```python
from build123d import *

# Parameters (mm, degrees)
F1_DEPTH = 5.588
F3_DEPTH = 7.62
F4_R     = 3.175
F5_DEPTH = 12.7
F6_R     = 1.27
F7_DEPTH = 8.128


with BuildPart() as f1:
    # F0 (on Front) → F1 (new body)
    with BuildSketch(Plane.XZ):
        with BuildLine():
            Line((12.7, -41.275), (12.7, 41.275))
            ThreePointArc((12.7, 41.275), (0, 53.975), (-12.7, 41.275))
            Line((-12.7, 41.275), (-12.7, -41.275))
            ThreePointArc((-12.7, -41.275), (0, -53.975), (12.7, -41.275))
        make_face()
    extrude(amount=F1_DEPTH)

    # F2 (on face) → F3 (join)
    with BuildSketch(Plane(origin=(0, 0, 0), x_dir=(-1, 0, 0), z_dir=(0, 1, 0))):
        with BuildLine():
            ThreePointArc((4.445, 34.3189235197), (7.2401139494, 37.309426271), (8.255, 41.275))
            ThreePointArc((8.255, 41.275), (-3.965573729, 48.5151139494), (-4.445, 34.3189235197))
            ThreePointArc((-4.445, 34.3189235197), (0, 33.02), (4.445, 34.3189235197))
        make_face()
        with BuildLine():
            ThreePointArc((4.445, 34.3189235197), (0, 33.02), (-4.445, 34.3189235197))
            Line((-4.445, 34.3189235197), (-4.445, 3.7810764803))
            ThreePointArc((-4.445, 3.7810764803), (0, 5.08), (4.445, 3.7810764803))
            Line((4.445, 3.7810764803), (4.445, 34.3189235197))
        make_face()
        with BuildLine():
            ThreePointArc((4.445, 3.7810764803), (0, 5.08), (-4.445, 3.7810764803))
            ThreePointArc((-4.445, 3.7810764803), (-8.2238434682, -3.89153584), (-3.175, -10.795))
            ThreePointArc((-3.175, -10.795), (0, -10.16), (3.175, -10.795))
            ThreePointArc((3.175, -10.795), (6.8685751798, -7.7540501198), (8.255, -3.175))
            ThreePointArc((8.255, -3.175), (7.2401139494, 0.790573729), (4.445, 3.7810764803))
        make_face()
        with BuildLine():
            ThreePointArc((3.175, -10.795), (0, -11.43), (-3.175, -10.795))
            ThreePointArc((-3.175, -10.795), (-8.2238434682, -17.69846416), (-4.445, -25.3710764803))
            ThreePointArc((-4.445, -25.3710764803), (0, -26.67), (4.445, -25.3710764803))
            ThreePointArc((4.445, -25.3710764803), (7.2401139494, -22.380573729), (8.255, -18.415))
            ThreePointArc((8.255, -18.415), (6.8685751798, -13.8359498802), (3.175, -10.795))
        make_face()
        with BuildLine():
            ThreePointArc((3.175, -10.795), (0, -10.16), (-3.175, -10.795))
            ThreePointArc((-3.175, -10.795), (0, -11.43), (3.175, -10.795))
        make_face()
        with BuildLine():
            ThreePointArc((4.445, -25.3710764803), (0, -26.67), (-4.445, -25.3710764803))
            Line((-4.445, -25.3710764803), (-4.445, -34.3189235197))
            ThreePointArc((-4.445, -34.3189235197), (0, -33.02), (4.445, -34.3189235197))
            Line((4.445, -34.3189235197), (4.445, -25.3710764803))
        make_face()
        with BuildLine():
            ThreePointArc((4.445, -34.3189235197), (0, -33.02), (-4.445, -34.3189235197))
            ThreePointArc((-4.445, -34.3189235197), (-3.965573729, -48.5151139494), (8.255, -41.275))
            ThreePointArc((8.255, -41.275), (7.2401139494, -37.309426271), (4.445, -34.3189235197))
        make_face()
    extrude(amount=F3_DEPTH)

    # F4 (on face) → F5 (join)
    with BuildSketch(Plane.XZ.offset(5.588)):
        with Locations((0, -41.275)):
            Circle(F4_R)
        with Locations((0, 41.275)):
            Circle(F4_R)
        with Locations((0, -3.175)):
            Circle(F4_R)
        with Locations((0, -18.415)):
            Circle(F4_R)
    extrude(amount=F5_DEPTH)

    # F6 (on face) → F7 (join)
    with BuildSketch(Plane.XZ.offset(18.288)):
        with Locations((0, 41.275)):
            Circle(F6_R)
        with Locations((0, -3.175)):
            Circle(F6_R)
        with Locations((0, -18.415)):
            Circle(F6_R)
        with Locations((0, -41.275)):
            Circle(F6_R)
    extrude(amount=F7_DEPTH)


solid = f1.part
```
Build history of the part. All positions in model axes, mm. A direction names the side the tool comes from. Give positions to 0.01 mm unless a question says otherwise; leave off trailing zeros. Loops run counter-clockwise (first coordinate to the right, second up) from the corner with the lowest first, then second, coordinate; pieces in that order, holes last.
1) Band-saw the part on D-D on y = -23. List the corners of the cut face in (x, z) (3 decimals), then the cut area to 3 significant figures.
Values follow:
outline: circle Ø2.54 at (0, -41.275); circle Ø2.54 at (0, -18.415); circle Ø2.54 at (0, -3.175); circle Ø2.54 at (0, 41.275)
area: 20.3 mm2
2) Band-saw the part on C-C on x = -10.25. List the corners of the cut face in (y, z), then the cut area to 3 significant figures.
Values follow:
outline: (-5.59, -48.77) - (0, -48.77) - (0, 48.77) - (-5.59, 48.77) - close
area: 545 mm2
3) Drop flat-ended pins along their axis: P1, Ø8.5, axis at y = 5, z = -29.5, coming from the +X side; P2, Ø6, axis at y = 5.5, z = 12, coming from the +X side (3 decimals); P3, Ø4, axis at y = 3.5, z = 14.5, coming from the -X side (3 decimals). Give the stop position or say it passes through.
Values follow:
P1: stops at x = 4.63
P2: stops at x = 4.445
P3: stops at x = -4.445
4) 3-axis set-ups, long thin cutter, end or side, ignore diameter. For faces 1 (the face through (-4.445, 4, 19)), 2 (the face through (0, -26.416, -41)), 3 (the face through (-0.275, -22.295, -42.515)), 4 (the face through (8, 0, 1)): which of +Z, -Z, +X, -X, +Y, -Y reach the whole face in a straight line?
Values follow:
face 1: -X, +Y
face 2: +Z, -Z, +X, -X, -Y
face 3: -Y
face 4: +Y
5) Two-plate mould, pull along Z, no slides. Class faces 5 (the face through (0.28, -2.75, 53.97)), 6 (the face through (-0.165, -22.295, 42.534)), 7 (the face through (0, 7.62, 1)): released by +Z, released by -Z, zero draft, split by the parting line, or undercut.
Values follow:
face 5: released by +Z
face 6: undercut
face 7: zero draft
6) Band-saw the part on B-B on y = -10.5. List the corners of the cut face in (x, z) (3 decimals), then the cut area to 3 significant figures.
Values follow:
outline: circle Ø6.35 at (0, -41.275); circle Ø6.35 at (0, -18.415); circle Ø6.35 at (0, -3.175); circle Ø6.35 at (0, 41.275)
area: 127 mm2
7) Probe line 1 along Y through (x, z) = (2.25, 34); line 2 along Y through (x, z) = (8, -32.5); line 3 along Z through (x, y) = (-7, 3). List the from-to ranges inside material, lowest first.
Values follow:
line 1: y = -5.59 to 7.62
line 2: y = -5.59 to 0
line 3: z = -45.65 to -36.9, -22.79 to -14.04, -7.55 to 1.2, 36.9 to 45.65
8) Band-saw the part on A-A on z = 17.5. List the corners of the cut face in (x, y) (3 decimals).
Values follow:
outline: (-12.7, -5.588) - (12.7, -5.588) - (12.7, 0) - (4.445, 0) - (4.445, 7.62) - (-4.445, 7.62) - (-4.445, 0) - (-12.7, 0) - close
